Could you check a few things on this drawing? It's one solid part, dimensions in mm from its lowest x, y, z. Give positions to 0.01 mm unless a question says otherwise; leave off trailing zeros. Write each loop counter-clockwise with the first axis right and the second up, starting at its lowest first coordinate (ties: lowest second). Pieces come first, ordered by that corner, then holes. Notation, with made-up numbers: M 21,58.25 L 57,58.25 A28 cw 57,79.25 Z; hole C 66.5,46 d4. An arc over 180 degrees is marked long. Write each question's results on one line, items separated by ' | '.
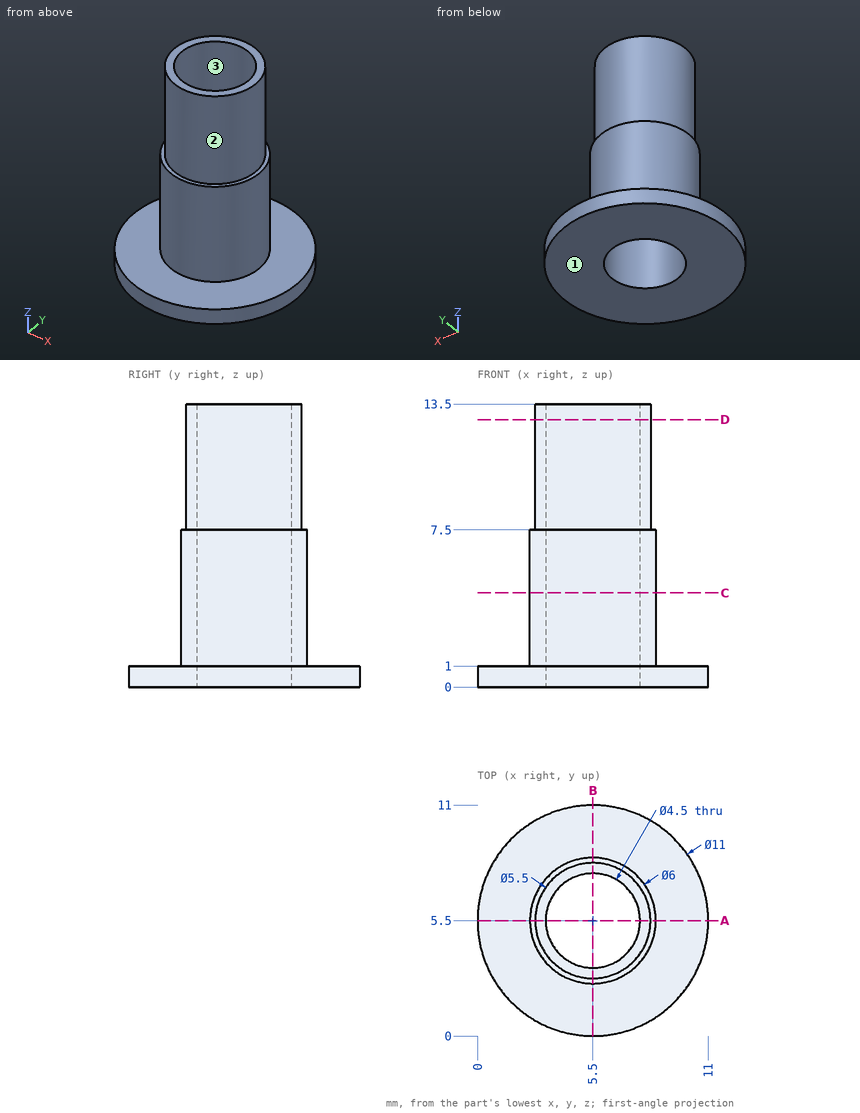
Item 1: I want a section at A-A, the plane y = 5.5. Please give me the cut outline in (x, z), and give its area (4 significant figures).
Geometry says:
outline: M 0,0 L 3.25,0 L 3.25,13.5 L 2.75,13.5 L 2.75,7.5 L 2.5,7.5 L 2.5,1 L 0,1 Z; M 7.75,0 L 11,0 L 11,1 L 8.5,1 L 8.5,7.5 L 8.25,7.5 L 8.25,13.5 L 7.75,13.5 Z | area: 22.25 mm2
Item 2: I want a section at C-C, the plane z = 4.5. Please give me the cut outline in (x, y), and give its area (3 significant figures).
Geometry says:
outline: C 5.5,5.5 d6; hole C 5.5,5.5 d4.5 | area: 12.4 mm2
Item 3: I'm going to push flat-ended pins straight in: pin 1 (4 mm diameter, centred on x = 5.5, z = 7, fed in from +Y); pin 2 (1 mm diameter, centred on x = 7.5, z = 9, fed in from +Y); pin 3 (1 mm diameter, centred on y = 4, z = 4.5, fed in from +X). Where does each tip first touch, or does it pass through?
Geometry says:
pin 1: stops at y = 8.5 | pin 2: stops at y = 7.8 | pin 3: stops at x = 8.33
Item 4: If I drill on line 1 (Y direction, x = 5.5, z = 10.25); line 2 (Y direction, x = 5.5, z = 6.75); line 3 (Z direction, x = 6.75, y = 0.5), over which ranges is the centre line in solid material (lowest first)? Write a range as from..to.
Geometry says:
line 1: y = 2.75..3.25, 7.75..8.25 | line 2: y = 2.5..3.25, 7.75..8.5 | line 3: z = 0..1
Item 5: Thinking about a two-plate mould opening in X: for the marked faces 1, 2 and 3, which applies, +X half, -X half, draft (parallel to the pull), parting line (faces both ways), or undercut?
Geometry says:
face 1: draft | face 2: parting line | face 3: undercut
Item 6: I want a section at D-D, the plane z = 12.75. Please give me the cut outline in (x, y).
Geometry says:
outline: C 5.5,5.5 d5.5; hole C 5.5,5.5 d4.5
